```python
from build123d import *

# Parameters (mm, degrees)
SKETCH1_R              = 3.3782
BOSS_EXTRUDE1_DEPTH    = 3.175
F_10_CLEARANCE_HOLE1_D = 5.1054
CHAMFER1_SIZE          = 3.175


with BuildPart() as part:
    # Sketch1 → Boss-Extrude1 (new body)
    with BuildSketch(Plane.XY):
        with BuildLine():
            Line((0, 0), (33.451477372, 0))
            ThreePointArc((33.451477372, 0), (37.816769242, 0.77380082), (41.650113644, 3.000909152))
            Line((41.650113644, 3.000909152), (63.298977204, 21.300681864))
            ThreePointArc((63.298977204, 21.300681864), (66.675, 28.575), (63.298977204, 35.849318136))
            Line((63.298977204, 35.849318136), (41.650113644, 54.149090848))
            ThreePointArc((41.650113644, 54.149090848), (37.816769242, 56.37619918), (33.451477372, 57.15))
            Line((33.451477372, 57.15), (0, 57.15))
            Line((0, 57.15), (0, 0))
        make_face()
        with Locations((57.15, 28.575)):
            Circle(SKETCH1_R, mode=Mode.SUBTRACT)
    extrude(amount=BOSS_EXTRUDE1_DEPTH)

    # #10 Clearance Hole1 (through all)
    with Locations(Plane.XY.offset(3.175)):
        with Locations((28.575, 28.575), (9.525, 28.575), (9.525, 47.625), (28.575, 47.625), (28.575, 9.525), (9.525, 9.525)):
            Hole(F_10_CLEARANCE_HOLE1_D / 2)

    # Chamfer1
    chamfer1_edges = [part.edges().sort_by_distance(p)[0] for p in [
        (0, 57.15, 1.5875),
        (0, 0, 1.5875),
    ]]
    chamfer(chamfer1_edges, length=CHAMFER1_SIZE)


solid = part.part
```
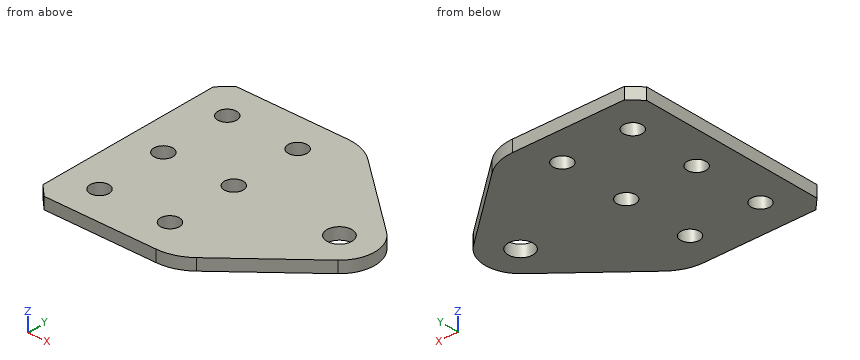
Check sheet for the modelled part. Datum: model origin and axes. Units: mm. Coordinates: 2 decimals unless noted, no trailing zeros. Order: outer loops, then holes, each group sorted by start corner. A loop starts at its lowest first (then second) coordinate and runs counter-clockwise, first axis right, second up. Notation, with made-up numbers: (88.5, 18) -> (122.5, 18) arc R26 cw to (122.5, 43) -> close; hole circle Ø11 at (49.25, 84.5). An arc over 180 degrees is marked (long way). Write each question's results on one line, items separated by ' | '. Start each with the question number.
1) Material ranges on line 1 along X through (y, z) = (29, 1.8); line 2 along Y through (x, z) = (28, 1.55); line 3 along Y through (x, z) = (8, 0.4), recorded low to high.
2) Section check C-C (x = 9). Enter the section's corners in (y, z) (3 decimals).
3) Depth check by flat-ended pin: pin 1 (3 mm diameter, centred on x = 9.525, y = 47.625, fed in from +Z). Enter the tip coordinate at first touch or a pass-through.
4) Section check B-B (y = 8). Enter the section's corners in (x, z) (3 decimals), and give its area (3 significant figures).
5) Section check D-D (z = 2). Enter the section's corners in (x, y) (3 decimals), and give its area (3 significant figures).
6) Section check A-A (x = 57.15). Enter the section's corners in (y, z) (3 decimals), and give its area (3 significant figures).
Checked values:
1) line 1: 0 to 7.01, 12.04 to 26.06, 31.09 to 53.8, 60.5 to 66.67 | line 2: 0 to 7.04, 12.01 to 26.09, 31.06 to 45.14, 50.11 to 57.15 | line 3: 0 to 7.48, 11.57 to 26.53, 30.62 to 45.58, 49.67 to 57.15
2) outline: (0, 0) -> (7.027, 0) -> (7.027, 3.175) -> (0, 3.175) -> close; (12.023, 0) -> (26.077, 0) -> (26.077, 3.175) -> (12.023, 3.175) -> close; (31.073, 0) -> (45.127, 0) -> (45.127, 3.175) -> (31.073, 3.175) -> close; (50.123, 0) -> (57.15, 0) -> (57.15, 3.175) -> (50.123, 3.175) -> close
3) pin 1: through
4) outline: (0, 0) -> (7.478, 0) -> (7.478, 3.175) -> (0, 3.175) -> close; (11.572, 0) -> (26.528, 0) -> (26.528, 3.175) -> (11.572, 3.175) -> close; (30.622, 0) -> (47.564, 0) -> (47.564, 3.175) -> (30.622, 3.175) -> close | area: 125 mm²
5) outline: (0, 3.175) -> (3.175, 0) -> (33.451, 0) arc R12.7 ccw to (41.65, 3.001) -> (63.299, 21.301) arc R9.525 ccw to (63.299, 35.849) -> (41.65, 54.149) arc R12.7 ccw to (33.451, 57.15) -> (3.175, 57.15) -> (0, 53.975) -> close; hole circle Ø5.105 at (9.525, 9.525); hole circle Ø5.105 at (9.525, 28.575); hole circle Ø5.105 at (9.525, 47.625); hole circle Ø5.105 at (28.575, 9.525); hole circle Ø5.105 at (28.575, 28.575); hole circle Ø5.105 at (28.575, 47.625); hole circle Ø6.756 at (57.15, 28.575) | area: 2,940 mm²
6) outline: (16.103, 0) -> (25.197, 0) -> (25.197, 3.175) -> (16.103, 3.175) -> close; (31.953, 0) -> (41.047, 0) -> (41.047, 3.175) -> (31.953, 3.175) -> close | area: 57.7 mm²
